from build123d import *

# Parameters (mm, degrees)
BOSS_EXTRU_1_DEPTH      = 10
ESQUISSE2_W             = 163.5
ESQUISSE2_H             = 109
ENL_V_MAT_EXTRU_1_DEPTH = 10
ESQUISSE3_W             = 164.5
ESQUISSE3_H             = 110
ENL_V_MAT_EXTRU_2_DEPTH = 8
ENL_V_MAT_EXTRU_3_DEPTH = 7
ESQUISSE5_R             = 3.5
BOSS_EXTRU_2_DEPTH      = 4
CONG_1_R                = 5
ESQUISSE6_W             = 12.13
ESQUISSE6_H             = 21
ESQUISSE6_W_2           = 8
ESQUISSE6_H_2           = 11
ENL_V_MAT_EXTRU_4_DEPTH = 97.5


# Read off the part's stored shape, not the designer's step: Fraisage pour vis à tête fraisée M31
with BuildPart() as part:
    # Esquisse1 → Boss.-Extru.1 (new body)
    with BuildSketch(Plane.XY):
        with BuildLine():
            Line((87.5, -75), (-87.5, -75))
            ThreePointArc((-87.5, -75), (-94.571067812, -72.071067812), (-97.5, -65))
            Line((-97.5, -65), (-97.5, 65))
            ThreePointArc((-97.5, 65), (-94.571067812, 72.071067812), (-87.5, 75))
            Line((-87.5, 75), (87.5, 75))
            ThreePointArc((87.5, 75), (94.571067812, 72.071067812), (97.5, 65))
            Line((97.5, 65), (97.5, -65))
            ThreePointArc((97.5, -65), (94.571067812, -72.071067812), (87.5, -75))
        make_face()
    extrude(amount=BOSS_EXTRU_1_DEPTH)

    # Esquisse2 → Enlèv. mat.-Extru.1 (cut)
    with BuildSketch(Plane.XY.offset(10)):
        with Locations((0, 2.25)):
            Rectangle(ESQUISSE2_W, ESQUISSE2_H)
    extrude(amount=-ENL_V_MAT_EXTRU_1_DEPTH, mode=Mode.SUBTRACT)

    # Esquisse3 → Enlèv. mat.-Extru.2 (cut)
    with BuildSketch(Plane(origin=(0, 0, 0), x_dir=(-1, 0, 0), z_dir=(0, 0, -1))):
        with Locations((0, 2.25)):
            Rectangle(ESQUISSE3_W, ESQUISSE3_H)
    extrude(amount=-ENL_V_MAT_EXTRU_2_DEPTH, mode=Mode.SUBTRACT)

    # Esquisse4 → Enlèv. mat.-Extru.3 (cut)
    with BuildSketch(Plane(origin=(0, 0, 0), x_dir=(-1, 0, 0), z_dir=(0, 0, -1))):
        with BuildLine():
            Line((-74.305753882, -63.01), (74.305753882, -63.01))
            ThreePointArc((74.305753882, -63.01), (78.51, -67.214246118), (82.714246118, -63.01))
            Line((82.714246118, -63.01), (82.714246118, 63.01))
            ThreePointArc((82.714246118, 63.01), (78.51, 67.214246118), (74.305753882, 63.01))
            Line((74.305753882, 63.01), (-74.305753882, 63.01))
            ThreePointArc((-74.305753882, 63.01), (-78.51, 67.214246118), (-82.714246118, 63.01))
            Line((-82.714246118, 63.01), (-82.714246118, -63.01))
            ThreePointArc((-82.714246118, -63.01), (-78.51, -67.214246118), (-74.305753882, -63.01))
        make_face()
    extrude(amount=-ENL_V_MAT_EXTRU_3_DEPTH, mode=Mode.SUBTRACT)

    # Esquisse5 → Boss.-Extru.2 (add)
    with BuildSketch(Plane(origin=(0, 0, 7), x_dir=(-1, 0, 0), z_dir=(0, 0, -1))):
        with Locations((-78.5, -62.75)):
            Circle(ESQUISSE5_R)
        with Locations((78.5, -62.75)):
            Circle(ESQUISSE5_R)
        with Locations((78.5, 62.75)):
            Circle(ESQUISSE5_R)
        with Locations((-78.5, 62.75)):
            Circle(ESQUISSE5_R)
    extrude(amount=BOSS_EXTRU_2_DEPTH)

    # Congé1
    cong_1_edges = [part.edges().sort_by_distance(p)[0] for p in [
        (-94.571067812, 72.071067812, 10),
        (-97.5, 0, 10),
        (-94.571067812, -72.071067812, 10),
        (0, -75, 10),
        (94.571067812, -72.071067812, 10),
        (97.5, 0, 10),
        (94.571067812, 72.071067812, 10),
        (0, 75, 10),
    ]]
    fillet(cong_1_edges, radius=CONG_1_R)

    # Esquisse6 → Enlèv. mat.-Extru.4 (cut)
    with BuildSketch(Plane(origin=(0, 0, 0), x_dir=(0, 0, -1), z_dir=(1, 0, 0))):
        with Locations((1.265, 46.5)):
            Rectangle(ESQUISSE6_W, ESQUISSE6_H)
        with Locations((-0.5, 19)):
            Rectangle(ESQUISSE6_W_2, ESQUISSE6_H_2)
        with Locations((-0.5, 5.5)):
            Rectangle(ESQUISSE6_W_2, ESQUISSE6_H_2)
    extrude(amount=ENL_V_MAT_EXTRU_4_DEPTH, mode=Mode.SUBTRACT)

    # Fraisage pour vis à tête fraisée M31 out → Fraisage pour vis à tête fraisée M31 (revolve, cut)
    with BuildSketch(Plane(origin=(-78.5, -62.75, 0), x_dir=(1, 0, 0), z_dir=(0, -1, 0))):
        Polygon((0, 3), (1.7, 3), (1.7, 8.05), (3.15, 9.5), (3.15, 10), (0, 10), align=None)
    revolve(axis=Axis((-78.5, -62.75, 0), (0, 0, 1)), mode=Mode.SUBTRACT)

    # Fraisage pour vis _ t_te frais_e M31 2 o → Fraisage pour vis _ t_te frais_e M31 2 (revolve, cut)
    with BuildSketch(Plane(origin=(78.5, -62.75, 0), x_dir=(1, 0, 0), z_dir=(0, -1, 0))):
        Polygon((0, 3), (1.7, 3), (1.7, 8.05), (3.15, 9.5), (3.15, 10), (0, 10), align=None)
    revolve(axis=Axis((78.5, -62.75, 0), (0, 0, 1)), mode=Mode.SUBTRACT)

    # Fraisage pour vis _ t_te frais_e M31 3 o → Fraisage pour vis _ t_te frais_e M31 3 (revolve, cut)
    with BuildSketch(Plane(origin=(78.5, 62.75, 0), x_dir=(1, 0, 0), z_dir=(0, -1, 0))):
        Polygon((0, 3), (1.7, 3), (1.7, 8.05), (3.15, 9.5), (3.15, 10), (0, 10), align=None)
    revolve(axis=Axis((78.5, 62.75, 0), (0, 0, 1)), mode=Mode.SUBTRACT)

    # Fraisage pour vis _ t_te frais_e M31 4 o → Fraisage pour vis _ t_te frais_e M31 4 (revolve, cut)
    with BuildSketch(Plane(origin=(-78.5, 62.75, 0), x_dir=(1, 0, 0), z_dir=(0, -1, 0))):
        Polygon((0, 3), (1.7, 3), (1.7, 8.05), (3.15, 9.5), (3.15, 10), (0, 10), align=None)
    revolve(axis=Axis((-78.5, 62.75, 0), (0, 0, 1)), mode=Mode.SUBTRACT)


solid = part.part
Work out the finished part from the listing and answer in its coordinate system (mm). A direction names the side the tool comes from. Round coordinates to 2 decimals unless told otherwise and drop trailing zeros. Write each loop counter-clockwise with the first axis right and the second up, starting at its lowest first coordinate (ties: lowest second). Pieces come first, ordered by that corner, then holes. Notation, with made-up numbers: (77.5, 62.5) - (134.5, 62.5) arc R32 cw to (134.5, 98.5) - close; hole circle Ø2 at (50, 41.5). An arc over 180 degrees is marked (long way). Answer in a Markdown table with one row per item. Add a question column.
1. Given pin 1 (4.5 mm diameter, centred on x = -78.5, y = -62.75, fed in from -Z); pin 2 (4 mm diameter, centred on x = 78.5, y = -62.75, fed in from +Z); pin 3 (1.4 mm diameter, centred on x = 89.5, z = 2.5, fed in from -Y), each flat-ended and moving along its own axis, determine where each tip first touches the part or whether it passes through.
2. A cutting plane is placed at C-C, the plane z = 1.5. Determine the outline of the cut face in (x, y).
3. A cutting plane is placed at A-A, the plane y = -49.5. Determine the outline of the cut face in (x, z).
4. A cutting plane is placed at B-B, the plane x = 9. Determine the outline of the cut face in (y, z), and give its area (3 significant figures).
5. For faces 5 (the cylindrical face through (-81.84, 63.8, 5.03)), 6 (the flat face through (90, 13.5, 2)), 7 (the flat face through (-14, -66, 0)), 8 (the cylindrical face through (-81, -64.667, 9.754)), 9 (the cylindrical face through (-94.49, -72.15, 2.47)), determine the directions among +Z, -Z, +X, -X, +Y, -Y from which every point of the face is accessible in a straight line to the end or side of a thin tool.
6. Find the intervals of material crossed by line 1 along Y through (x, z) = (30, 3); line 2 along X through (y, z) = (-57.5, 1); line 3 along Z through (x, y) = (-12.5, 57), in increasing order. Write a range as from..to.
7. The mould has two halves that part along Y. Classify faces 1 (the cylindrical face through (1, 73, 9)), 2 (the cylindrical face through (-96, 0.91, 8.57)), 3 (the cylindrical face through (94.65, -71.99, 2.47)), 4 (the cylindrical face through (76, 60.833, 9.754)): +Y half, -Y half, draft (parallel to the pull), parting line (faces both ways), or undercut.
Worked out:
| question | item | result |
|---|---|---|
| 1 | pin 1 | z = 3 |
| 1 | pin 2 | z = 8.35 |
| 1 | pin 3 | y = -74.92 |
| 2 | outline | (-97.5, -65) arc R10 ccw to (-87.5, -75) - (87.5, -75) arc R10 ccw to (97.5, -65) - (97.5, 0) - (82.71, 0) - (82.71, -63.01) arc R4.2 cw to (74.31, -63.01) - (-74.31, -63.01) arc R4.2 cw to (-82.71, -63.01) - (-82.71, 63.01) arc R4.2 cw to (-74.31, 63.01) - (74.31, 63.01) arc R4.2 cw to (82.71, 63.01) - (82.71, 57) - (97.5, 57) - (97.5, 65) arc R10 ccw to (87.5, 75) - (-87.5, 75) arc R10 ccw to (-97.5, 65) - close; (82.71, 11) - (97.5, 11) - (97.5, 13.5) - (82.71, 13.5) - close; (82.71, 24.5) - (97.5, 24.5) - (97.5, 36) - (82.71, 36) - close |
| 3 | outline | (-97.5, 0) - (-82.71, 0) - (-82.71, 7) - (-82.25, 7) - (-82.25, 8) - (-81.75, 8) - (-81.75, 10) - (-92.5, 10) arc R5 ccw to (-97.5, 5) - close; (81.75, 8) - (82.25, 8) - (82.25, 7) - (82.71, 7) - (82.71, 0) - (97.5, 0) - (97.5, 5) arc R5 ccw to (92.5, 10) - (81.75, 10) - close |
| 4 | outline | (-75, 0) - (-63.01, 0) - (-63.01, 7) - (-52.75, 7) - (-52.75, 8) - (-52.25, 8) - (-52.25, 10) - (-70, 10) arc R5 ccw to (-75, 5) - close; (56.75, 8) - (57.25, 8) - (57.25, 7) - (63.01, 7) - (63.01, 0) - (75, 0) - (75, 5) arc R5 ccw to (70, 10) - (56.75, 10) - close |
| 4 | area | 279 mm^2 |
| 5 | face 5 | -Z |
| 5 | face 6 | -Z, +X |
| 5 | face 7 | -Z, +X, -X, +Y, -Y |
| 5 | face 8 | +Z |
| 5 | face 9 | +Z, -Z, -X, -Y |
| 6 | line 1 | -75..-63.01, 63.01..75 |
| 6 | line 2 | -97.5..-82.71, 82.71..97.5 |
| 6 | line 3 | 8..10 |
| 7 | face 1 | +Y half |
| 7 | face 2 | draft |
| 7 | face 3 | -Y half |
| 7 | face 4 | undercut |
